Could you check a few things on this model? Use its own coordinates, in mm. Round coordinates to 2 decimals unless told otherwise and drop trailing zeros. Loops run counter-clockwise (first coordinate to the right, second up) from the corner with the lowest first, then second, coordinate; pieces in that order, holes last. Notation, with made-up numbers: (-6, 18.5) -> (42, 18.5) arc R27 ccw to (42, 47.5) -> close; hole circle Ø9 at (2, 24). An arc over 180 degrees is marked (long way). One line per item, written item: value.
from build123d import *

# Parameters (mm, degrees)
F0_W     = 228.6
F0_H     = 152.4
F1_DEPTH = 76.2
F3_DEPTH = 152.4
F4_R     = 5.08
F5_R     = 3.81
F6_DEPTH = 6.35
F7_DEPTH = 5.08


with BuildPart() as f1:
    # F0 (on Top) → F1 (new body)
    with BuildSketch(Plane.XY):
        Rectangle(F0_W, F0_H)
    extrude(amount=F1_DEPTH)

    # F2 (on face) → F3 (cut)
    with BuildSketch(Plane.XZ.offset(76.2)):
        Polygon((-114.3, 76.2), (-114.3, 0), (114.3, 76.2), align=None)
    extrude(amount=-F3_DEPTH, mode=Mode.SUBTRACT)

    # F4
    f4_edges = [f1.edges().sort_by_distance(p)[0] for p in [
        (-114.3, 0, 0),
        (114.3, 0, 76.2),
        (0, -76.2, 38.1),
        (0, 76.2, 38.1),
        (114.3, -76.2, 38.1),
        (114.3, 76.2, 38.1),
        (114.3, 0, 0),
        (0, 76.2, 0),
        (0, -76.2, 0),
    ]]
    fillet(f4_edges, radius=F4_R)

    # F5 (on face) → F6 (cut)
    with BuildSketch(Plane(origin=(-11.43, 0, 34.29), x_dir=(0.9486832981, 0, 0.316227766), z_dir=(-0.316227766, 0, 0.9486832981))):
        with Locations((105.6566610932, -51.5762679279)):
            Circle(F5_R)
        with Locations((105.6566610932, 51.5762679279)):
            Circle(F5_R)
        with Locations((24.1764013898, 0)):
            Circle(F5_R)
        with Locations((-57.3038583136, 51.5762679279)):
            Circle(F5_R)
        with Locations((-57.3038583136, -51.5762679279)):
            Circle(F5_R)
    extrude(amount=-F6_DEPTH, mode=Mode.SUBTRACT)

    # F7 (cut): a face of the model
    f7_faces = [f1.faces().sort_by_distance(p)[0] for p in [
        (-82.2535384016, 0, 10.6821538661),
    ]]
    extrude(f7_faces, amount=-F7_DEPTH, mode=Mode.SUBTRACT)


solid = f1.part
(1) I'm going to push flat-ended pins straight in: pin 1 Ø1.5 at (x, y) = (-41, 52.5) entering from +Z; pin 2 Ø20.5 at (x, z) = (-25.5, 42) entering from +Y. Where does each tip first touch, or does it pass through?
Recorded:
pin 1: z = 19.33
pin 2: through
(2) If I drill on L1, parallel to Y at x = 16.5, z = 37.5; L2, parallel to Y at x = 88, z = 64.5; L3, parallel to Z at x = 1, y = -30, over which ranges is the centre line in solid material (lowest first)?
Recorded:
L1: -76.2 to -1.84, 1.84 to 76.2
L2: -75.65 to -71.12, 71.12 to 75.65
L3: 0 to 33.08
(3) Thinking about a two-plate mould opening in Y: for faces 1 (the face through (87.945, 54.151, 61.4)), 2 (the face through (14.458, 74.672, 1.449)), 3 (the face through (12, 1, 0)), which applies, released by +Y, released by -Y, zero draft, split by the parting line, or undercut?
Recorded:
face 1: undercut
face 2: released by +Y
face 3: zero draft
(4) If we section it at A-A, the plane y = 16.5: Please give me the cut outline in (x, z), then the cut area to 3 significant figures.
Recorded:
outline: (-84.6, 9.9) arc R5.08 ccw to (-83, 0) -> (109.22, 0) arc R5.08 ccw to (114.3, 5.08) -> (114.3, 69.15) arc R5.08 ccw to (107.61, 73.97) -> (109.22, 69.15) -> (-83, 5.08) -> close
area: 7,540 mm²
